Study the drawing (mm; zero at the part's minimum x, y, z) and answer. Coordinates: 2 decimals unless noted, no trailing zeros. Order: outer loops, then holes, each group sorted by start corner. A loop starts at its lowest first (then second) coordinate and runs counter-clockwise, first axis right, second up. Notation, with made-up numbers: M 25.5,13.5 L 70.5,13.5 A27 ccw 70.5,46.5 Z; hole C -32.5,12 d7. An arc over 180 degrees is marked long. One line per item, written item: value. Start each with the question number.
Q1. Straight lines are drawn through the part: line 1 along Y through (x, z) = (30, 1.1); line 2 along Y through (x, z) = (54, 1.15) (1 decimal); line 3 along X through (y, z) = (3, 2.55). For each, find the intervals that lie inside material, in ascending order. Write a range as [from, to].
Q2. The part is cut by section A-A on x = 32. Give the vertices of the cut face in (y, z).
Q3. Each of these flat-tipped pins is pushed along its axis until it touches: pin 1 Ø1.2 at (x, z) = (78.5, 1.5) entering from -Y; pin 2 Ø1 at (y, z) = (31, 1) entering from -X; pin 3 Ø1.2 at (x, z) = (23.5, 2.5) entering from +Y; pin 4 Ø1.2 at (x, z) = (28.5, 2) entering from -Y. Where does it stop, or does it pass through?
Q4. The part is cut by section C-C on z = 3.4. Give the vertices of the cut face in (x, y) (1 decimal), then the cut area to 4 significant figures.
Q5. The part is cut by section B-B on y = 15.5. Give the vertices of the cut face in (x, z) (1 decimal).
Q6. The part is cut by section D-D on y = 10. Give the vertices of the cut face in (x, z), then the cut area to 3 significant figures.
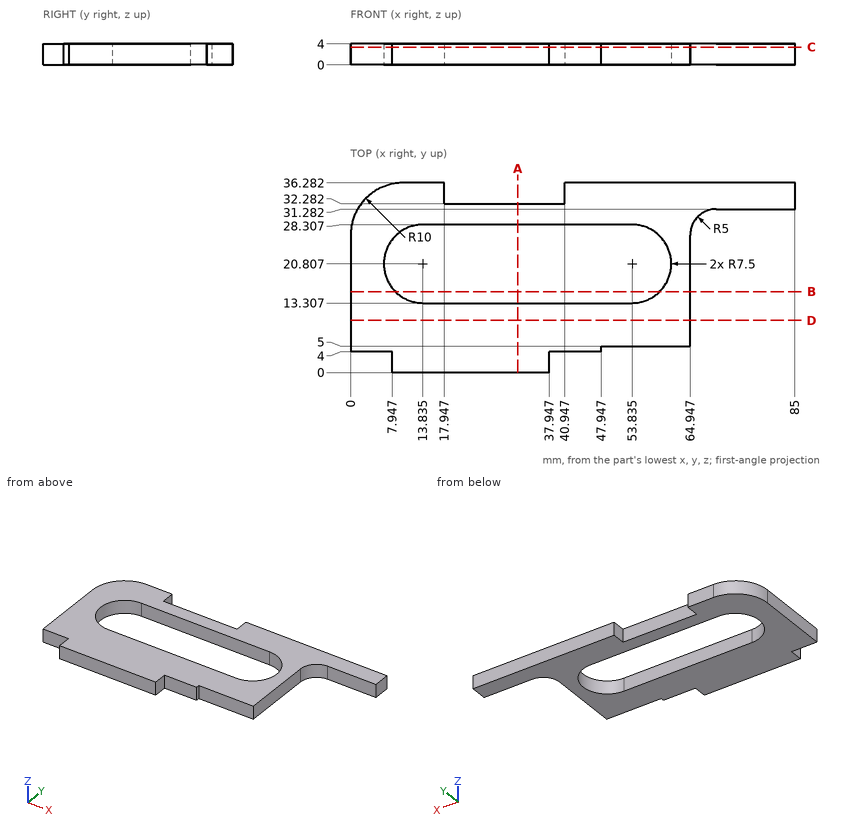
Output:
1. line 1: y = [0, 13.31], [28.31, 32.28]
1. line 2: y = [5, 13.3], [28.3, 36.3]
1. line 3: x = [7.95, 37.95]
2. outline: M 0,0 L 13.31,0 L 13.31,4 L 0,4 Z; M 28.31,0 L 32.28,0 L 32.28,4 L 28.31,4 Z
3. pin 1: stops at y = 31.28
3. pin 2: stops at x = 0.93
3. pin 3: stops at y = 32.28
3. pin 4: stops at y = 0
4. outline: M 0,4 L 7.9,4 L 7.9,0 L 37.9,0 L 37.9,4 L 47.9,4 L 47.9,5 L 64.9,5 L 64.9,26.3 A5 cw 69.9,31.3 L 85,31.3 L 85,36.3 L 40.9,36.3 L 40.9,32.3 L 17.9,32.3 L 17.9,36.3 L 10,36.3 A10 ccw 0,26.3 Z; hole M 13.8,13.3 L 53.8,13.3 A7.5 ccw 53.8,28.3 L 13.8,28.3 A7.5 ccw Z
4. area: 1,415 mm^2
5. outline: M 0,0 L 8.5,0 L 8.5,4 L 0,4 Z; M 59.1,0 L 64.9,0 L 64.9,4 L 59.1,4 Z
6. outline: M 0,0 L 64.95,0 L 64.95,4 L 0,4 Z
6. area: 260 mm^2
